The model under review builds one solid part; all positions refer to its coordinate system, in mm. A direction names the side the tool comes from. Coordinates: 2 decimals unless noted, no trailing zeros. Loops run counter-clockwise (first coordinate to the right, second up) from the corner with the lowest first, then second, coordinate; pieces in that order, holes last. Notation, with made-up numbers: (15.5, 0.25) - (39.5, 0.25) arc R32 cw to (39.5, 34.25) - close; hole circle Ø6 at (31.25, 73). An arc over 180 degrees is marked (long way). Use a Markdown table: item, result. Add a question column.
1) The part is to be moulded in two halves that separate along X. For faces 4 (the flat face through (8, 37, -25)), 5 (the flat face through (30, 14.3, -14.9)), 6 (the flat face through (0, 14.3, -14.9)), 7 (the cylindrical face through (9.28, 23.77, -25.44)), say which applies: pulls with the +X half, pulls with the -X half, needs draft (parallel to the pull), parting line crosses it, or undercut.
2) For faces 1 (the flat face through (14.8, 0, -0.4)), 2 (the flat face through (15, 7, -0.9)), 3 (the flat face through (15, 15, -13)), list the 3-axis set-ups (+Z, -Z, +X, -X, +Y, -Y) from which the entire face can be reached by the end or side of a thin tool; tool diameter is ignored.
3) Add section B-B, the plane y = 30. Give the boundary of the cut face in (x, z), and give its area (3 significant figures).
4) Add section D-D, the plane y = 7.5. Give the boundary of the cut face in (x, z), and give its area (3 significant figures).
5) To check wall thickness, follow L1, parallel to X at y = 30, z = -25.55; L2, parallel to Z at x = 10.25, y = 37.5; L3, parallel to Y at x = 6.25, z = -22.75. State the ranges of each line that lie inside material, in increasing order. Write a range as [from, to].
6) Clearance check with flat-ended pins moving along their axes: pin 1 (6.5 mm diameter, centred on x = 18.5, z = -16.5, fed in from -Y); pin 2 (14.5 mm diameter, centred on x = 8, y = 33.5, fed in from +Z); pin 3 (6.5 mm diameter, centred on x = 18, z = -16.5, fed in from +Y). State where each tip first meets the part, or that it passes through.
7) Add section A-A, the plane x = 15. Give the boundary of the cut face in (y, z).
8) Add section C-C, the plane z = -5. Give the boundary of the cut face in (x, y), and give its area (3 significant figures).
Autodesk Inventor part; units mm, degrees
ref_plane "YZ Plane" through (0, 0, 0) normal (1, 0, 0) x (0, 1, 0)
ref_plane "XZ Plane" through (0, 0, 0) normal (0, 1, 0) x (-1, 0, 0)
ref_plane "XY Plane" through (0, 0, 0) normal (0, 0, 1) x (1, 0, 0)
sketch "Sketch1" plane through (0, 0, 0) normal (0, 0, 1) x (1, 0, 0)
  line L0 (0, 0) -> (30, 0)
  line L1 (30, 0) -> (30, 15)
  line L2 (30, 15) -> (0, 15)
  line L3 (0, 15) -> (0, 0)
  dimension "d0" = 15
  dimension "d1" = 30
extrude "Plate1" add sketch "Sketch1" against normal blind 0.9
sketch "Sketch2" plane through (30, 14.1, 0) normal (0, 1, 0) x (-1, 0, 0)
  line L0 (30, 0) -> (0, 0)
  line L1 (0, 0) -> (0, -25.9)
  line L2 (0, -25.9) -> (30, -25.9)
  line L3 (30, -25.9) -> (30, 0)
edge flange "Flange1" height 25.9 angle 90 thickness 0.9 bend radius 0.9 thickness toward (0, 1, 0) relief tear relief width 0.9 relief depth 0.45 edges at (15, 15, -0.9) wall of the first edge with corners at (0, 14.1, 0) (30, 14.1, 0) (30, 14.1, -25.9) (0, 14.1, -25.9)
bend "Bend1"
corner "Corner1"
sketch "Sketch3" plane through (0, 14.1, -25) normal (0, 0, -1) x (-1, 0, 0)
  line L0 (-30, 0) -> (0, 0)
  line L1 (0, 0) -> (0, 30.9)
  line L2 (0, 30.9) -> (-30, 30.9)
  line L3 (-30, 30.9) -> (-30, 0)
edge flange "Flange2" height 30.9 angle 90 thickness 0.9 bend radius 0.9 thickness toward (0, 0, -1) relief tear relief width 0.9 relief depth 0.45 edges at (15, 15, -25.9) wall of the first edge with corners at (30, 14.1, -25) (0, 14.1, -25) (0, 45, -25) (30, 45, -25)
bend "Bend2"
corner "Corner2"
sketch "Sketch4" plane through (30, 45, -25.9) normal (0, 0, -1) x (-1, 0, 0)
  line L0 (30, 0) -> (30, -29.1)
  line L1 (0, 0) -> (30, 0)
  point P0 (30, -45)
  point P1 (15, -15)
  dimension "d23" = 15
  dimension "d24" = 15
hole "Hole1" at (15, 30, -25.9) direction (0, 0, 1) diameter 16.9175 end through all
equation "\"d2\" = Thickness"
equation "\"d3\" = BendReliefWidth"
equation "\"d4\" = BendReliefDepth"
equation "\"d5\" = MinimumRemnant"
equation "\"d6\" = TransitionRadius"
equation "\"d9\" = BendRadius"
equation "\"d10\" = CornerReliefSize"
equation "\"d11\" = GapSize"
equation "\"d12\" = JacobiRadiusSize"
equation "\"d13\" = BendReliefWidth"
equation "\"d14\" = BendReliefDepth"
equation "\"d15\" = MinimumRemnant"
equation "\"d16\" = TransitionRadius"
equation "\"d19\" = BendRadius"
equation "\"d20\" = CornerReliefSize"
equation "\"d21\" = GapSize"
equation "\"d22\" = JacobiRadiusSize"
equation "\"BendRadius\" = Thickness"
equation "\"BendReliefWidth\" = Thickness"
equation "\"BendReliefDepth\" = 0.5 * Thickness"
equation "\"CornerReliefSize\" = 4 * Thickness"
equation "\"MinimumRemnant\" = 2 * Thickness"
equation "\"TransitionRadius\" = BendRadius"
equation "\"JacobiRadiusSize\" = BendRadius"
equation "\"GapSize\" = Thickness"
properties part number "Soporte Sensor Inductivo"
From the geometry:
| question | item | result |
|---|---|---|
| 1 | face 4 | needs draft |
| 1 | face 5 | pulls with the +X half |
| 1 | face 6 | pulls with the -X half |
| 1 | face 7 | undercut |
| 2 | face 1 | +Z, -Z, +X, -X, -Y |
| 2 | face 2 | -Z, +X, -X, -Y |
| 2 | face 3 | +Z, +X, -X, +Y |
| 3 | outline | (0, -25.9) - (6.54, -25.9) - (6.54, -25) - (0, -25) - close; (23.46, -25.9) - (30, -25.9) - (30, -25) - (23.46, -25) - close |
| 3 | area | 11.8 mm^2 |
| 4 | outline | (0, -0.9) - (30, -0.9) - (30, 0) - (0, 0) - close |
| 4 | area | 27.0 mm^2 |
| 5 | L1 | x = [0, 6.54], [23.46, 30] |
| 5 | L2 | z = [-25.9, -25] |
| 5 | L3 | y = [14.1, 15] |
| 6 | pin 1 | stops at y = 14.1 |
| 6 | pin 2 | stops at z = -25 |
| 6 | pin 3 | stops at y = 15 |
| 7 | outline | (0, -0.9) - (13.2, -0.9) arc R0.9 cw to (14.1, -1.8) - (14.1, -24.1) arc R1.8 ccw to (15.9, -25.9) - (21.54, -25.9) - (21.54, -25) - (15.9, -25) arc R0.9 cw to (15, -24.1) - (15, -1.8) arc R1.8 ccw to (13.2, 0) - (0, 0) - close; (38.46, -25.9) - (45, -25.9) - (45, -25) - (38.46, -25) - close |
| 8 | outline | (0, 14.1) - (30, 14.1) - (30, 15) - (0, 15) - close |
| 8 | area | 27.0 mm^2 |
